Geometry check sheet. Reference: drawing and pictorial views, mm from the part's lowest x, y, z. Give positions to 0.01 mm unless a question says otherwise; leave off trailing zeros. Write each loop counter-clockwise with the first axis right and the second up, starting at its lowest first coordinate (ties: lowest second). Pieces come first, ordered by that corner, then holes. Notation, with made-up numbers: (-29, 68.25) -> (7, 68.25) arc R15 cw to (7, 86.25) -> close; hole circle Ø2 at (-30, -39.5). An arc over 180 degrees is marked (long way). Answer as CSV lines item,"result".
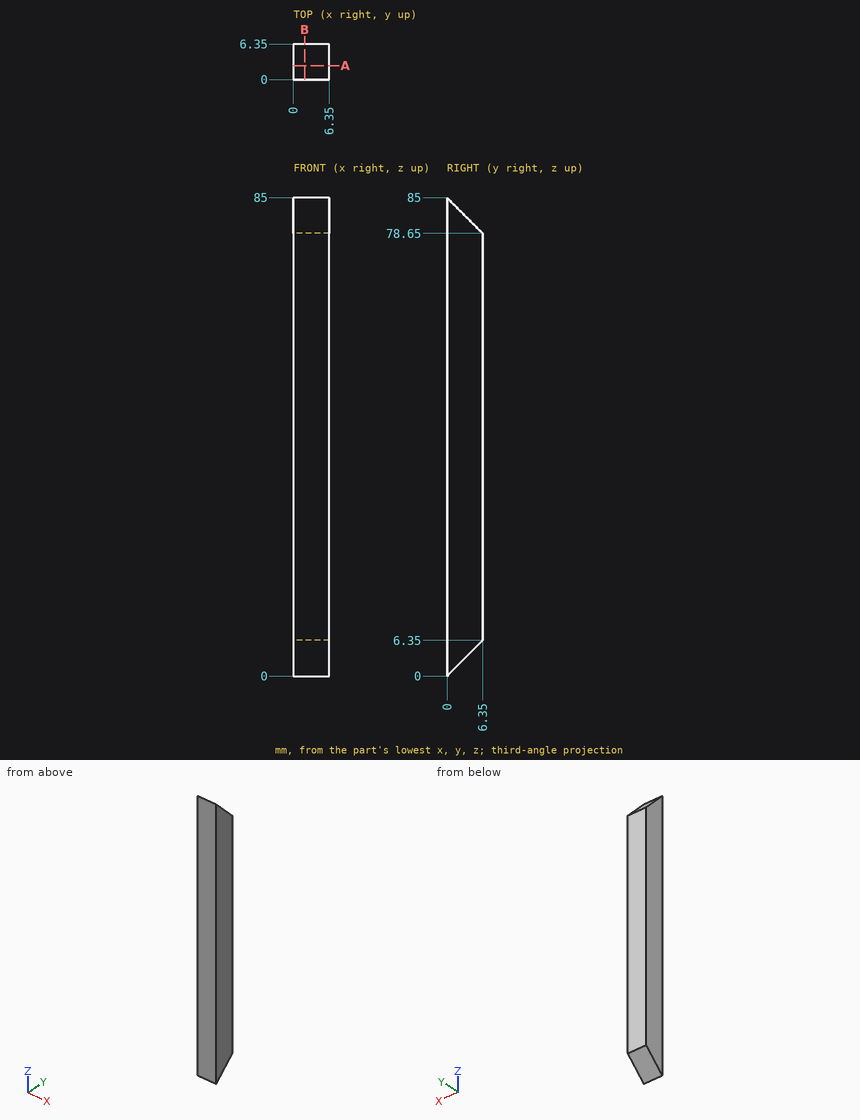
1) Section check B-B (x = 2). Record the boundary of the cut face in (y, z).
Reported:
outline,"(0, 0) -> (6.35, 6.35) -> (6.35, 78.65) -> (0, 85) -> close"
2) Scan lines: line 1 along Z through (x, y) = (4.5, 6); line 2 along Z through (x, y) = (4.5, 4). Record each from-to range of solid material in increasing order.
Reported:
line 1,"6 to 79"
line 2,"4 to 81"
3) Section check A-A (y = 2.5). Record the boundary of the cut face in (x, z), and give its area (3 significant figures).
Reported:
outline,"(0, 2.5) -> (6.35, 2.5) -> (6.35, 82.5) -> (0, 82.5) -> close"
area,"508 mm²"
